from build123d import *

# Parameters (mm, degrees)
F1_DEPTH       = 5.08
F2_SIZE        = 2.54
F4_D           = 3.6576
F4_START       = 0.635
F4_START_2     = 0.6350001
F4_CBORE_D     = 6.35
F4_CBORE_DEPTH = 3.5052
F5_W           = 32.0675
F5_H           = 184.15
F6_DEPTH       = 5.081
F7_W           = 32.0675
F7_H           = 184.15
F8_DEPTH       = 3.2766


with BuildPart() as f1:
    # F0 (on Front) → F1 (new body)
    with BuildSketch(Plane.XZ):
        with BuildLine():
            ThreePointArc((26.19375, 96.52), (24.7058524484, 100.1121024484), (21.11375, 101.6))
            Line((21.11375, 101.6), (-21.11375, 101.6))
            ThreePointArc((-21.11375, 101.6), (-24.7058524484, 100.1121024484), (-26.19375, 96.52))
            Line((-26.19375, 96.52), (-26.19375, -96.52))
            ThreePointArc((-26.19375, -96.52), (-24.7058524484, -100.1121024484), (-21.11375, -101.6))
            Line((-21.11375, -101.6), (21.11375, -101.6))
            ThreePointArc((21.11375, -101.6), (24.7058524484, -100.1121024484), (26.19375, -96.52))
            Line((26.19375, -96.52), (26.19375, 96.52))
        make_face()
    extrude(amount=F1_DEPTH)

    # F2
    f2_edges = [f1.edges().sort_by_distance(p)[0] for p in [
        (0, -5.08, 101.6),
    ]]
    chamfer(f2_edges, length=F2_SIZE)

    # F4 (through all)
    # its depths count from where the whole tool has entered the part; down to there all is cleared
    with Locations(Plane.XZ.offset(5.08)):
        with Locations((-21.11375, 96.52, -F4_START_2), (21.11375, 96.52, -F4_START_2), (21.11375, 0, -F4_START), (-21.11375, 0, -F4_START), (-21.11375, -96.52, -F4_START_2), (21.11375, -96.52, -F4_START_2)):
            CounterBoreHole(F4_D / 2, F4_CBORE_D / 2, F4_CBORE_DEPTH)

    # F5 (on face) → F6 (cut, through all)
    with BuildSketch(Plane.XZ.offset(5.08)):
        Rectangle(F5_W, F5_H)
    extrude(amount=-F6_DEPTH, mode=Mode.SUBTRACT)

    # F7 (on face) → F8 (cut)
    with BuildSketch(Plane(origin=(0, 0, 0), x_dir=(-1, 0, 0), z_dir=(0, 1, 0))):
        with BuildLine():
            ThreePointArc((21.11375, 90.17), (16.6236219395, 92.0298719395), (14.76375, 96.52))
            Line((14.76375, 96.52), (-14.76375, 96.52))
            ThreePointArc((-14.76375, 96.52), (-16.6236219395, 92.0298719395), (-21.11375, 90.17))
            Line((-21.11375, 90.17), (-21.11375, 4.445))
            ThreePointArc((-21.11375, 4.445), (-16.66875, 0), (-21.11375, -4.445))
            Line((-21.11375, -4.445), (-21.11375, -90.17))
            ThreePointArc((-21.11375, -90.17), (-16.6236219395, -92.0298719395), (-14.76375, -96.52))
            Line((-14.76375, -96.52), (14.76375, -96.52))
            ThreePointArc((14.76375, -96.52), (16.6236219395, -92.0298719395), (21.11375, -90.17))
            Line((21.11375, -90.17), (21.11375, -4.445))
            ThreePointArc((21.11375, -4.445), (16.66875, 0), (21.11375, 4.445))
            Line((21.11375, 4.445), (21.11375, 90.17))
        make_face()
        Rectangle(F7_W, F7_H, mode=Mode.SUBTRACT)
    extrude(amount=-F8_DEPTH, mode=Mode.SUBTRACT)


solid = f1.part
Check sheet for the modelled part. Datum: model origin and axes. Units: mm. A direction names the side the tool comes from. Round coordinates to 2 decimals unless told otherwise and drop trailing zeros. Order: outer loops, then holes, each group sorted by start corner. A loop starts at its lowest first (then second) coordinate and runs counter-clockwise, first axis right, second up.
Q1. Cross-section at C-C, the plane z = 0. Enter the section's corners in (x, y) (3 decimals), plus the area to 3 significant figures.
Filled sheet:
outline: (-26.194, -2.54) - (-24.289, -4.445) - (-24.289, -0.94) - (-22.943, -0.94) - (-22.943, 0) - (-26.194, 0) - close; (-19.285, -0.94) - (-17.939, -0.94) - (-17.939, -5.08) - (-16.034, -5.08) - (-16.034, -3.277) - (-16.669, -3.277) - (-16.669, 0) - (-19.285, 0) - close; (16.034, -5.08) - (17.939, -5.08) - (17.939, -0.94) - (19.285, -0.94) - (19.285, 0) - (16.669, 0) - (16.669, -3.277) - (16.034, -3.277) - close; (22.943, -0.94) - (24.289, -0.94) - (24.289, -4.445) - (26.194, -2.54) - (26.194, 0) - (22.943, 0) - close
area: 33.6 mm2
Q2. Cross-section at B-B, the plane z = 64. Enter the section's corners in (x, y), plus the area to 3 significant figures.
Filled sheet:
outline: (-26.19, -2.54) - (-23.65, -5.08) - (-16.03, -5.08) - (-16.03, -3.28) - (-21.11, -3.28) - (-21.11, 0) - (-26.19, 0) - close; (16.03, -5.08) - (23.65, -5.08) - (26.19, -2.54) - (26.19, 0) - (21.11, 0) - (21.11, -3.28) - (16.03, -3.28) - close
area: 63.5 mm2
Q3. Set-up check for faces 4 (the face through (-18, -5.08, 15)), 5 (the face through (-16.575, -1.615, -92.08)), 6 (the face through (23.2, -0.94, -96.5)): record each of +Z, -Z, +X, -X, +Y, -Y from which the full face is reachable in a straight line by a thin tool's end or side.
Filled sheet:
face 4: +Z, -Z, +X, -X, -Y
face 5: +Y
face 6: -Y
Q4. Cross-section at A-A, the plane x = 0.5. Enter the section's corners in (y, z) (3 decimals), plus the area to 3 significant figures.
Filled sheet:
outline: (-5.08, -99.06) - (-2.54, -101.6) - (0, -101.6) - (0, -96.52) - (-3.277, -96.52) - (-3.277, -92.075) - (-5.08, -92.075) - close; (-5.08, 92.075) - (-3.277, 92.075) - (-3.277, 96.52) - (0, 96.52) - (0, 101.6) - (-2.54, 101.6) - (-5.08, 99.06) - close
area: 61.2 mm2
Q5. Depth check by flat-ended pin: P1, Ø2, axis at x = 14, z = 53, coming from the -Y side; P2, Ø4, axis at x = -21.11, z = 96.52, coming from the -Y side; P3, Ø0.5, axis at y = -4.5, z = 42, coming from the +X side; P4, Ø1.4, axis at x = 3.5, y = -4, coming from the +Z side. Enter the tip coordinate at first touch or a pass-through.
Filled sheet:
P1: passes through
P2: stops at y = -0.94
P3: stops at x = 24.48
P4: stops at z = 100.84
Q6. Draft check along X on faces 1 (the face through (24.75, -1.25, 100.07)), 2 (the face through (-18, 0, 0)), 3 (the face through (23.2, -0.94, 96.6)). Enter one of: pulls with the +X half, pulls with the -X half, needs draft (parallel to the pull), parting line crosses it, or undercut.
Filled sheet:
face 1: pulls with the +X half
face 2: needs draft
face 3: undercut
Q7. Scan lines: L1, parallel to Z at x = 4, y = -1.8; L2, parallel to X at y = -1.7, z = 70; L3, parallel to Z at x = -23, y = -3.8. Record each from-to range of solid material in increasing order.
Filled sheet:
L1: z = -101.6 to -96.52, 96.52 to 101.6
L2: x = -26.19 to -21.11, 21.11 to 26.19
L3: z = -99.84 to -99.07, -93.97 to -2.55, 2.55 to 93.97, 99.07 to 99.84
